```python
from build123d import *

# Parameters (mm, degrees)
F0_W     = 49
F0_H     = 25.5652221807
F1_DEPTH = 12
F2_W     = 29
F2_H     = 21.5
F3_DEPTH = 2
F4_W     = 25
F4_H     = 17.5
F5_DEPTH = 12
F7_D     = 3.2639
F8_R     = 1.207
F9_R     = 1.207
F10_R    = 1.207
F11_R    = 1.207


# Not quite as in the source:
# - a feature names something its author has since deleted; it is built from what else it names


with BuildPart() as f1:
    # F0 (on Top) → F1 (new body)
    with BuildSketch(Plane.XY):
        Rectangle(F0_W, F0_H)
    extrude(amount=-F1_DEPTH)

    # F2 (on face) → F3 (cut)
    with BuildSketch(Plane.XY):
        Rectangle(F2_W, F2_H)
    extrude(amount=-F3_DEPTH, mode=Mode.SUBTRACT)

    # F4 (on Top) → F5 (cut)
    with BuildSketch(Plane.XY):
        Rectangle(F4_W, F4_H)
    extrude(amount=-F5_DEPTH, mode=Mode.SUBTRACT)

    # F7 (through all)
    with Locations(Plane.XY):
        with Locations((-19.5, 0), (19.5, 0)):
            Hole(F7_D / 2)

    # F8
    f8_edges = [f1.edges().sort_by_distance(p)[0] for p in [
        (0, -12.782611, 0),
    ]]
    fillet(f8_edges, radius=F8_R)

    # F9
    f9_edges = [f1.edges().sort_by_distance(p)[0] for p in [
        (24.5, 0.6035, 0),
    ]]
    fillet(f9_edges, radius=F9_R)

    # F10
    f10_edges = [f1.edges().sort_by_distance(p)[0] for p in [
        (-24.5, 0.6035, 0),
    ]]
    fillet(f10_edges, radius=F10_R)

    # F11
    f11_edges = [f1.edges().sort_by_distance(p)[0] for p in [
        (0, 12.782611, 0),
    ]]
    fillet(f11_edges, radius=F11_R)


solid = f1.part
```
Here's how the part is built. I have some questions about the finished solid (model axes, mm). A direction names the side the tool comes from. Coordinates: 2 decimals unless noted, no trailing zeros. Order: outer loops, then holes, each group sorted by start corner. A loop starts at its lowest first (then second) coordinate and runs counter-clockwise, first axis right, second up.
1) I need wall thicknesses on line 1 (X direction, y = 4.5, z = -9); line 2 (Y direction, x = -19.5, z = -6.5); line 3 (Y direction, x = 9, z = -7). Which ranges of each line are inside material? Lowest first, please.
2) Imagine slicing it at C-C on y = -6.75. List the corners of the cut face in (x, z) for me, and give its area (3 significant figures).
3) Which directions (+Z, -Z, +X, -X, +Y, -Y) give clear straight access to the entire face, cutting with the end or side of a thin tool? Please do faces 4 (the face through (0, 8.75, -7)), 5 (the face through (-24.156, 0.162, -0.363)), 6 (the face through (0, 10.75, -1)).
4) Imagine slicing it at B-B on x = -19.5. List the corners of the cut face in (y, z) for me.
5) Will these pins go through, and if not, where does the flat tip stop? pin 1 (8 mm diameter, centred on x = -9.5, y = 8.5, fed in from -Z); pin 2 (1.5 mm diameter, centred on x = -9, y = 9.5, fed in from +Z).
6) Imagine slicing it at D-D on z = -10.5. List the corners of the cut face in (x, y) for me, and give its area (3 significant figures).
7) We'd pull the mould along Y, two halves only. Please class faces 1 (the face through (-24.5, 0, -7)), 2 (the face through (14.5, 0, -1)), 3 (the face through (0, -12.783, -7)): +Y half, -Y half, draft (parallel to the pull), parting line (faces both ways), or undercut.
8) Imagine slicing it at A-A on y = 0. List the corners of the cut face in (x, z) for me.
Response values:
1. line 1: x = -24.5 to -12.5, 12.5 to 24.5
1. line 2: y = -12.78 to -1.63, 1.63 to 12.78
1. line 3: y = -12.78 to -8.75, 8.75 to 12.78
2. outline: (-24.5, -12) - (-12.5, -12) - (-12.5, -2) - (-14.5, -2) - (-14.5, 0) - (-23.29, 0) arc R1.21 ccw to (-24.5, -1.21) - close; (12.5, -12) - (24.5, -12) - (24.5, -1.21) arc R1.21 ccw to (23.29, 0) - (14.5, 0) - (14.5, -2) - (12.5, -2) - close
2. area: 279 mm2
3. face 4: +Z, -Z
3. face 5: +Z, -X, +Y, -Y
3. face 6: +Z
4. outline: (-12.78, -12) - (-1.63, -12) - (-1.63, 0) - (-11.58, 0) arc R1.21 ccw to (-12.78, -1.21) - close; (1.63, -12) - (12.78, -12) - (12.78, -1.21) arc R1.21 ccw to (11.58, 0) - (1.63, 0) - close
5. pin 1: stops at z = -12
5. pin 2: stops at z = -2
6. outline: (-24.5, -11.58) arc R1.21 ccw to (-23.29, -12.78) - (23.29, -12.78) arc R1.21 ccw to (24.5, -11.58) - (24.5, 11.58) arc R1.21 ccw to (23.29, 12.78) - (-23.29, 12.78) arc R1.21 ccw to (-24.5, 11.58) - close; hole circle Ø3.26 at (-19.5, 0); hole (-12.5, -8.75) - (12.5, -8.75) - (12.5, 8.75) - (-12.5, 8.75) - close; hole circle Ø3.26 at (19.5, 0)
6. area: 797 mm2
7. face 1: draft
7. face 2: undercut
7. face 3: -Y half
8. outline: (-24.5, -12) - (-21.13, -12) - (-21.13, 0) - (-23.29, 0) arc R1.21 ccw to (-24.5, -1.21) - close; (-17.87, -12) - (-12.5, -12) - (-12.5, -2) - (-14.5, -2) - (-14.5, 0) - (-17.87, 0) - close; (12.5, -12) - (17.87, -12) - (17.87, 0) - (14.5, 0) - (14.5, -2) - (12.5, -2) - close; (21.13, -12) - (24.5, -12) - (24.5, -1.21) arc R1.21 ccw to (23.29, 0) - (21.13, 0) - close
